Input: part model. Units: mm. Frame: model coordinates. A direction names the side the tool comes from. Coordinates: 2 decimals unless noted, no trailing zeros. Order: outer loops, then holes, each group sorted by start corner. A loop starts at its lowest first (then second) coordinate and runs counter-clockwise, first axis right, second up. Notation, with made-up numbers: (5, 61.5) -> (60, 61.5) arc R17 ccw to (60, 89.5) -> close; hole circle Ø11 at (43.5, -4). An arc over 180 degrees is marked (long way). One line per item, written item: value. Start each with the question number.
from build123d import *

# Parameters (mm, degrees)
SKETCH1_R                  = 4.5
BOSS_EXTRUDE1_DEPTH        = 6.35
BOSS_EXTRUDE1_2_DEPTH      = 6.35
BOSS_EXTRUDE2_DEPTH        = 3.175
SKETCH5_W                  = 4.5
SKETCH5_H                  = 3.175
BOSS_EXTRUDE3_DEPTH        = 11.43
F_6_CLEARANCE_HOLE1_D      = 3.7973
FILLET1_R                  = 2.54
FILLET2_R                  = 3.81
FILLET3_R                  = 12.7
CUT_EXTRUDE1_REACH         = 111.936
SKETCH10_R                 = 5.715
F_6_CLEARANCE_HOLE2_REACH  = 143.713
F_6_CLEARANCE_HOLE2_BORE_R = 1.89865
BOSS_EXTRUDE5_START        = 1.912
SKETCH13_R                 = 4.43865
SKETCH13_R_2               = 1.89865
BOSS_EXTRUDE5_DEPTH        = 1.912


with BuildPart() as part:
    # Sketch1 → Boss-Extrude1 (new body)
    with BuildSketch(Plane(origin=(0, 0, 0), x_dir=(1, 0, 0), z_dir=(0, 1, 0))):
        with Locations(Location((78.74, 0, 0), (0, 0, 270))):
            Circle(SKETCH1_R)
    extrude(amount=BOSS_EXTRUDE1_DEPTH)



with BuildPart() as body_2:
    # Sketch1 → Boss-Extrude1 2 (new body)
    with BuildSketch(Plane(origin=(0, 0, 0), x_dir=(1, 0, 0), z_dir=(0, 1, 0))):
        with Locations(Location((-78.74, 22.86, 0), (0, 0, 270))):
            Circle(SKETCH1_R)
    extrude(amount=BOSS_EXTRUDE1_2_DEPTH)


with BuildPart() as part_1:
    add(part.part)

    add(body_2.part)  # Boss-Extrude2 merges body 2
    # Sketch2 → Boss-Extrude2 (add)
    with BuildSketch(Plane(origin=(0, 0, 0), x_dir=(1, 0, 0), z_dir=(0, 1, 0))):
        with BuildLine():
            ThreePointArc((-74.24, 22.86), (-78.74, 18.36), (-83.24, 22.86))
            Line((-83.24, 22.86), (-83.24, -4.5))
            Line((-83.24, -4.5), (78.74, -4.5))
            ThreePointArc((78.74, -4.5), (74.24, 0), (78.74, 4.5))
            Line((78.74, 4.5), (-74.24, 4.5))
            Line((-74.24, 4.5), (-74.24, 22.86))
        make_face()
    extrude(amount=BOSS_EXTRUDE2_DEPTH)

    # Sketch5 → Boss-Extrude3 (add, symmetric)
    with BuildSketch(Plane.XY):
        with BuildLine():
            ThreePointArc((-90.114084776, 3.175), (-87.371075104, 22.291795245), (-80.620096155, 40.386))
            Line((-80.620096155, 40.386), (-87.664596069, 40.386))
            ThreePointArc((-87.664596069, 40.386), (-94.280160195, 20.672730678), (-96.52, 0))
            Line((-96.52, 0), (-83.24, 0))
            Line((-83.24, 0), (-83.24, 3.175))
            Line((-83.24, 3.175), (-90.114084776, 3.175))
        make_face()
        with BuildLine():
            Line((80.620096155, 40.386), (87.664596069, 40.386))
            ThreePointArc((87.664596069, 40.386), (86.567546752, 42.686886152), (85.41012022, 44.958))
            Line((85.41012022, 44.958), (78.162696576, 44.958))
            ThreePointArc((78.162696576, 44.958), (79.424301148, 42.689685958), (80.620096155, 40.386))
        make_face()
        with BuildLine():
            Line((-87.664596069, 40.386), (-80.620096155, 40.386))
            ThreePointArc((-80.620096155, 40.386), (-79.424301148, 42.689685958), (-78.162696576, 44.958))
            Line((-78.162696576, 44.958), (-85.41012022, 44.958))
            ThreePointArc((-85.41012022, 44.958), (-86.567546752, 42.686886152), (-87.664596069, 40.386))
        make_face()
        with BuildLine():
            Line((-80.620096155, 40.386), (80.620096155, 40.386))
            ThreePointArc((80.620096155, 40.386), (79.424301148, 42.689685958), (78.162696576, 44.958))
            Line((78.162696576, 44.958), (-78.162696576, 44.958))
            ThreePointArc((-78.162696576, 44.958), (-79.424301148, 42.689685958), (-80.620096155, 40.386))
        make_face()
        with Locations((80.99, 1.5875)):
            Rectangle(SKETCH5_W, SKETCH5_H)
        with BuildLine():
            Line((83.24, 3.175), (83.24, 0))
            Line((83.24, 0), (96.52, 0))
            ThreePointArc((96.52, 0), (94.280160195, 20.672730678), (87.664596069, 40.386))
            Line((87.664596069, 40.386), (80.620096155, 40.386))
            ThreePointArc((80.620096155, 40.386), (87.371075104, 22.291795245), (90.114084776, 3.175))
            Line((90.114084776, 3.175), (83.24, 3.175))
        make_face()
    extrude(amount=BOSS_EXTRUDE3_DEPTH, both=True)

    # #6 Clearance Hole1 (through all)
    with Locations(Plane(origin=(-78.74, 0, -22.86), x_dir=(0, 0, -1), z_dir=(0, -1, 0))):
        with Locations((0, 0), (-22.86, 157.48)):
            Hole(F_6_CLEARANCE_HOLE1_D / 2)

    # Fillet1
    fillet1_edges = [part_1.edges().sort_by_distance(p)[0] for p in [
        (-90.114084776, 3.175, 0),
        (90.114084776, 3.175, 0),
    ]]
    fillet(fillet1_edges, radius=FILLET1_R)

    # Fillet2
    # the kernel refuses this fillet: 3.81 mm, written as the material it adds along each edge
    with BuildSketch(Plane(origin=(80.620096155, 40.386, 5.835732073), x_dir=(-1, 0, 0), z_dir=(0, 0, -1))) as fillet2_piece_1_section:
        with BuildLine():
            CenterArc((2.388096155, -3.81), FILLET2_R, 90, 64.942384582)
            ThreePointArc((-1.06331561, -2.196352941), (-0.539087936, -1.094579337), (0, 0))
            Line((0, 0), (2.388096155, 0))
        make_face()
    fillet2_piece_1 = extrude(amount=17.265732073, mode=Mode.PRIVATE)
    fillet2_piece_1 = fillet2_piece_1 - Plane(origin=(78.74, 40.386, 0), x_dir=(0, 0, 1), z_dir=(0, 1, 0)) * Cylinder(1.89865, 45, mode=Mode.PRIVATE)
    add(fillet2_piece_1)
    with BuildSketch(Plane(origin=(80.620096155, 40.386, 11.43), x_dir=(-1, 0, 0), z_dir=(0, 0, -1))) as fillet2_piece_2_section:
        with BuildLine():
            CenterArc((2.388096155, -3.81), FILLET2_R, 90, 64.942384582)
            ThreePointArc((-1.06331561, -2.196352941), (-0.539087936, -1.094579337), (0, 0))
            Line((0, 0), (2.388096155, 0))
        make_face()
    fillet2_piece_2 = extrude(amount=17.265732073, mode=Mode.PRIVATE)
    fillet2_piece_2 = fillet2_piece_2 - Plane(origin=(78.74, 40.386, 0), x_dir=(0, 0, 1), z_dir=(0, 1, 0)) * Cylinder(1.89865, 45, mode=Mode.PRIVATE)
    add(fillet2_piece_2)
    with BuildSketch(Plane(origin=(-80.620096155, 40.386, -11.43), x_dir=(-0.4357482606496553, -0.900068582576239, 0), z_dir=(0, 0, 1))) as fillet2_piece_3:
        with BuildLine():
            CenterArc((2.388652554, 3.809651194), FILLET2_R, 205.832916425, 64.942384582)
            Line((-1.040608746, 2.149450321), (0, 0))
            ThreePointArc((0, 0), (1.220103103, -0.008255072), (2.440206206, 0))
        make_face()
    extrude(amount=22.86)
    # the kernel refuses this fillet: 3.81 mm, written as the material it takes off along each edge
    with BuildSketch(Plane(origin=(-85.41012022, 44.958, -17.378402089), x_dir=(-0.4548470974381097, -0.8905695469485393, 0), z_dir=(0, 0, 1))) as fillet2_2_piece_1:
        with BuildLine():
            CenterArc((2.332399766, 3.809710574), FILLET2_R, 207.055096642, 63.651134119)
            Line((-1.060670207, 2.076743133), (0, 0))
            ThreePointArc((0, 0), (1.189680418, -0.007332124), (2.379360836, 0))
        make_face()
    extrude(amount=34.756804178, mode=Mode.SUBTRACT)
    with BuildSketch(Plane(origin=(85.41012022, 44.958, 17.378402089), x_dir=(-1, 0, 0), z_dir=(0, 0, -1))) as fillet2_2_piece_2:
        with BuildLine():
            CenterArc((2.331926956, -3.81), FILLET2_R, 90, 63.651134119)
            ThreePointArc((-1.08224537, -2.118986301), (-0.547652451, -1.056158155), (0, 0))
            Line((0, 0), (2.331926956, 0))
        make_face()
    extrude(amount=34.756804178, mode=Mode.SUBTRACT)

    # Fillet3
    # the kernel refuses this fillet: 12.7 mm, written as the material it adds along each edge
    with BuildSketch(Plane(origin=(78.74, 0, -4.5), x_dir=(0, 0, -1), z_dir=(0, 1, 0)), Plane(origin=(-83.24, 0, 4.5), x_dir=(0, 0, 1), z_dir=(0, 1, 0))) as fillet3_piece_1:
        with BuildLine():
            CenterArc((12.7, 11.313580335), FILLET3_R, 180, 62.978120887)
            Line((0, 11.313580335), (0, 0))
            Line((0, 0), (6.93, 0))
        make_face()
    extrude(amount=3.175)
    with BuildSketch(Plane(origin=(78.74, 0, 4.5), x_dir=(0, 0, 1), z_dir=(0, 1, 0))) as fillet3_piece_2:
        with BuildLine():
            CenterArc((12.7, -11.313580335), FILLET3_R, 117.021879113, 62.978120887)
            Line((0, -11.313580335), (0, 0))
            Line((0, 0), (6.93, 0))
        make_face()
    extrude(amount=3.175)
    with BuildSketch(Plane(origin=(-74.24, 0, -4.5), x_dir=(1, 0, 0), z_dir=(0, 1, 0))) as fillet3_piece_3:
        with BuildLine():
            CenterArc((FILLET3_R, FILLET3_R), FILLET3_R, 180, 90)
            Line((0, FILLET3_R), (0, 0))
            Line((0, 0), (FILLET3_R, 0))
        make_face()
    extrude(amount=3.175)
    with BuildSketch(Plane(origin=(-83.24, 0, -11.43), x_dir=(-1, 0, 0), z_dir=(0, 1, 0))) as fillet3_piece_4:
        with BuildLine():
            CenterArc((12.636340451, -12.7), FILLET3_R, 90, 84.260829523)
            Line((0, -11.43), (0, 0))
            Line((0, 0), (12.636340451, 0))
        make_face()
    extrude(amount=3.175)

    # Cut-Extrude1: up to this face of the body (flat: up to its plane)
    cut_extrude1_end = Plane(part_1.part.faces().sort_by_distance((78.74, 6.35, -4.372720779))[0])
    # Sketch10 → Cut-Extrude1 (cut, up to the picked face)
    with BuildSketch(Plane(origin=(0, 44.958, 0), x_dir=(1, 0, 0), z_dir=(0, 1, 0)), mode=Mode.PRIVATE) as cut_extrude1_sk1:
        with Locations(Location((78.74, 0, 0), (0, 0, 95.099688914))):
            Circle(SKETCH10_R)
    cut_extrude1_tool1 = split(extrude(cut_extrude1_sk1.sketch, amount=-CUT_EXTRUDE1_REACH, mode=Mode.PRIVATE), bisect_by=cut_extrude1_end, keep=Keep.BOTH, mode=Mode.PRIVATE)
    add(cut_extrude1_tool1.solids().sort_by(Axis((78.74, 44.958, 0), (0, -1, 0)))[0], mode=Mode.SUBTRACT)

    # #6 Clearance Hole2 bore (on position points) → #6 Clearance Hole2 (cut, up to next)
    with BuildSketch(Plane(origin=(-33.5265, 44.958, 6.5405), x_dir=(1, 0, 0), z_dir=(0, 1, 0)), mode=Mode.PRIVATE) as f_6_clearance_hole2_sk1:
        Circle(F_6_CLEARANCE_HOLE2_BORE_R)
    f_6_clearance_hole2_tool1 = extrude(f_6_clearance_hole2_sk1.sketch, amount=-F_6_CLEARANCE_HOLE2_REACH, mode=Mode.PRIVATE) & part_1.part
    # #6 Clearance Hole2 bore (on position points) → #6 Clearance Hole2 (cut, up to next)
    with BuildSketch(Plane(origin=(-33.5265, 44.958, 6.5405), x_dir=(1, 0, 0), z_dir=(0, 1, 0)), mode=Mode.PRIVATE) as f_6_clearance_hole2_sk2:
        with Locations((98.3488, 2.286)):
            Circle(F_6_CLEARANCE_HOLE2_BORE_R)
    f_6_clearance_hole2_tool2 = extrude(f_6_clearance_hole2_sk2.sketch, amount=-F_6_CLEARANCE_HOLE2_REACH, mode=Mode.PRIVATE) & part_1.part
    add(f_6_clearance_hole2_tool1.solids().sort_by_distance((-33.5265, 44.958, 6.5405))[0], mode=Mode.SUBTRACT)
    add(f_6_clearance_hole2_tool2.solids().sort_by_distance((64.8223, 44.958, 4.2545))[0], mode=Mode.SUBTRACT)

    # Sketch13 → Boss-Extrude5 (add)
    # profile 1 of 2: a face of its own
    with BuildSketch(Plane(origin=(0, 44.958, 0), x_dir=(1, 0, 0), z_dir=(0, 1, 0)).offset(BOSS_EXTRUDE5_START)):
        with Locations(Location((-33.5265, -6.5405, 0), (0, 0, 180))):
            Circle(SKETCH13_R)
        with Locations(Location((-33.5265, -6.5405, 0), (0, 0, 180))):
            Circle(SKETCH13_R_2, mode=Mode.SUBTRACT)
    # profile 2 of 2: a face of its own
    with BuildSketch(Plane(origin=(0, 44.958, 0), x_dir=(1, 0, 0), z_dir=(0, 1, 0)).offset(BOSS_EXTRUDE5_START)):
        with Locations(Location((64.8223, -4.2545, 0), (0, 0, 180))):
            Circle(SKETCH13_R)
        with Locations(Location((64.8223, -4.2545, 0), (0, 0, 180))):
            Circle(SKETCH13_R_2, mode=Mode.SUBTRACT)
    extrude(amount=-BOSS_EXTRUDE5_DEPTH)


solid = part_1.part
1) Mould query, pull axis Y, two halves, no side actions, for faces 4 (the flat face through (-11, 3.175, -2)), 5 (the flat face through (-8, 0, -2)), 6 (the cylindrical face through (60.59, 45.93, 5.59)), 7 (the flat face through (-35.4, 46.87, 5.6)). Classes: +Y half, -Y half, draft (parallel to the pull), parting line (faces both ways), or undercut.
2) Section query C-C, the plane y = 36. Return the cut outline in (x, z) (3 decimals), plus the area to 3 significant figures.
3) Section query B-B, the plane y = 11. Return the cut outline in (x, z).
4) Ray query, line 1 along Z through (x, y) = (-78.74, 5.25); line 2 along Y through (x, z) = (2, -1.5) (3 decimals); line 3 along X through (y, z) = (4.25, 0). Return the intervals inside material, ascending. Write a range as from..to.
5) Pin query (flat end, axial travel): pin 1 Ø2.5 at (x, z) = (-33.53, 6.54) entering from +Y; pin 2 Ø1.5 at (x, z) = (-6.5, 7) entering from +Y; pin 3 Ø1.6 at (x, y) = (5.5, 1.5) entering from +Z; pin 4 Ø10 at (x, z) = (-81, -21) entering from +Y. Return the tip coordinate at first contact, or that it passes through.
6) Access query for faces 1 (the cylindrical face through (73.98, 1.57, -6.32)), 2 (the flat face through (-74.24, 2, -20)), 3 (the cylindrical face through (-78.542, 3.836, -27.356)). Directions: +Z, -Z, +X, -X, +Y, -Y. A direction counts if a zero-diameter tool reaches every point of the face in a straight line with its end or side. Return the directions, or none.
7) Section query A-A, the plane y = 22. Return the cut outline in (x, z) (3 decimals).
Entries:
1. face 4: undercut
1. face 5: -Y half
1. face 6: draft
1. face 7: +Y half
2. outline: (-89.555, -11.43) -> (-82.672, -11.43) -> (-82.672, 11.43) -> (-89.555, 11.43) -> close; (82.672, -11.43) -> (89.555, -11.43) -> (89.555, 11.43) -> (82.672, 11.43) -> (82.672, 4.148) arc R5.715 cw to (82.672, -4.148) -> close
2. area: 304 mm2
3. outline: (-95.89, -11.43) -> (-89.5, -11.43) -> (-89.5, 11.43) -> (-95.89, 11.43) -> close; (89.5, -11.43) -> (95.89, -11.43) -> (95.89, 11.43) -> (89.5, 11.43) -> close
4. line 1: z = -27.36..-24.76, -20.96..-18.36
4. line 2: y = 0..3.175, 40.386..44.958
4. line 3: x = -96.43..-89.52, 74.24..76.84, 80.64..83.24, 89.52..96.43
5. pin 1: passes through
5. pin 2: stops at y = 44.96
5. pin 3: stops at z = 4.5
5. pin 4: stops at y = 6.35
6. face 1: -Z, -Y
6. face 2: -Z, +X, +Y, -Y
6. face 3: +Y
7. outline: (-93.979, -11.43) -> (-87.445, -11.43) -> (-87.445, 11.43) -> (-93.979, 11.43) -> close; (87.445, -11.43) -> (93.979, -11.43) -> (93.979, 11.43) -> (87.445, 11.43) -> close
